from build123d import *

# Parameters (mm, degrees)
BOX007_W     = 7
BOX007_H     = 4
BOX007_DEPTH = 6
BOX002_W     = 30.1
BOX002_H     = 23.1
BOX002_DEPTH = 4
BOX003_W     = 12
BOX003_H     = 7
BOX003_DEPTH = 10
BOX001_W     = 40
BOX001_H     = 3
BOX001_DEPTH = 12
BOX004_W     = 4
BOX004_H     = 4
BOX004_DEPTH = 6
BOX005_W     = 4
BOX005_H     = 4
BOX005_DEPTH = 6
BOX008_W     = 30
BOX008_H     = 30
BOX008_DEPTH = 3
BOX006_W     = 19
BOX006_H     = 4
BOX006_DEPTH = 5


with BuildPart() as cube007:
    # Box007 → Box007 (new body)
    with BuildSketch(Plane(origin=(25, 1, 3), x_dir=(1, 0, 0), z_dir=(0, 0, 1))):
        with Locations((3.5, 2)):
            Rectangle(BOX007_W, BOX007_H)
    extrude(amount=BOX007_DEPTH)


with BuildPart() as cube002:
    # Box002 → Box002 (new body)
    with BuildSketch(Plane(origin=(7, 1, 3), x_dir=(1, 0, 0), z_dir=(0, 0, 1))):
        with Locations((15.05, 11.55)):
            Rectangle(BOX002_W, BOX002_H)
    extrude(amount=BOX002_DEPTH)


with BuildPart() as cube003:
    # Box003 → Box003 (new body)
    with BuildSketch(Plane(origin=(13, -4, 1), x_dir=(1, 0, 0), z_dir=(0, 0, 1))):
        with Locations((6, 3.5)):
            Rectangle(BOX003_W, BOX003_H)
    extrude(amount=BOX003_DEPTH)


with BuildPart() as cube001:
    # Box001 → Box001 (new body)
    with BuildSketch(Plane.XY):
        with Locations((20, 1.5)):
            Rectangle(BOX001_W, BOX001_H)
    extrude(amount=BOX001_DEPTH)


with BuildPart() as cube004:
    # Box004 → Box004 (new body)
    with BuildSketch(Plane(origin=(23, 22, 3), x_dir=(1, 0, 0), z_dir=(0, 0, 1))):
        with Locations((2, 2)):
            Rectangle(BOX004_W, BOX004_H)
    extrude(amount=BOX004_DEPTH)


with BuildPart() as cube005:
    # Box005 → Box005 (new body)
    with BuildSketch(Plane(origin=(4, 22, 3), x_dir=(1, 0, 0), z_dir=(0, 0, 1))):
        with Locations((2, 2)):
            Rectangle(BOX005_W, BOX005_H)
    extrude(amount=BOX005_DEPTH)


with BuildPart() as cut001:
    # Box008 → Box008 (new body)
    with BuildSketch(Plane.XY):
        with Locations((15, 15)):
            Rectangle(BOX008_W, BOX008_H)
    extrude(amount=BOX008_DEPTH)

    # Fusion001: union Cube001, Cube004, Cube005
    add(cube001.part)
    add(cube004.part)
    add(cube005.part)

    # Cut: cut Cube003
    add(cube003.part, mode=Mode.SUBTRACT)

    # Cut001: cut Cube002
    add(cube002.part, mode=Mode.SUBTRACT)


with BuildPart() as obj1:
    # Box006 → Box006 (new body)
    with BuildSketch(Plane(origin=(7, 1, 0), x_dir=(1, 0, 0), z_dir=(0, 0, 1))):
        with Locations((9.5, 2)):
            Rectangle(BOX006_W, BOX006_H)
    extrude(amount=BOX006_DEPTH)

    # Fusion002: union Cut001
    add(cut001.part)

    # Cut002: cut Cube007
    add(cube007.part, mode=Mode.SUBTRACT)


with BuildPart() as obj1_1:
    # Cut002 placement: moved
    add(obj1.part.moved(Location((113, -95, 26.4))))


solid = obj1_1.part
Read the model definition and answer for the solid it produces. Units are mm, in the model's axes. A direction names the side the tool comes from. Give positions to 0.01 mm unless a question says otherwise; leave off trailing zeros. Loops run counter-clockwise (first coordinate to the right, second up) from the corner with the lowest first, then second, coordinate; pieces in that order, holes last. Notation, with made-up numbers: (10.5, 70) -> (64.5, 70) arc R4 ccw to (64.5, 74) -> close; hole circle Ø4 at (34, -28). An arc over 180 degrees is marked (long way). Use a Markdown table: item, result.
Q1. Each of these flat-tipped pins is pushed along its axis until it touches: pin 1 (1.2 mm diameter, centred on y = -71.5, z = 32, fed in from -X); pin 2 (1 mm diameter, centred on x = 123, z = 32.5, fed in from +Y); pin 3 (4 mm diameter, centred on y = -88, z = 33, fed in from -X); pin 4 (3 mm diameter, centred on x = 134, z = 29.5, fed in from -Y). Where does it stop, or does it pass through?
Solved:
| item | result |
|---|---|
| pin 1 | stops at x = 117 |
| pin 2 | stops at y = -94 |
| pin 3 | passes through |
| pin 4 | stops at y = -94 |
Q2. Section A-A, the plane x = 130.5 is taken. Determine the outline of the cut face in (y, z).
Solved:
| item | result |
|---|---|
| outline | (-95, 26.4) -> (-65, 26.4) -> (-65, 29.4) -> (-90, 29.4) -> (-90, 31.4) -> (-94, 31.4) -> (-94, 27.4) -> (-95, 27.4) -> close; (-95, 37.4) -> (-92, 37.4) -> (-92, 38.4) -> (-95, 38.4) -> close |
Q3. A tool of negligible diameter and unlimited length cuts with its end or side. For faces 5 (the face through (141, -93, 35.4)), 6 (the face through (138, -69, 32)), 7 (the face through (148, -93, 33.4)), from which of +Z, -Z, +X, -X, +Y, -Y can it reach the whole face along a straight path? Write none if from no direction.
Solved:
| item | result |
|---|---|
| face 5 | none |
| face 6 | +Z, +X, -X, +Y |
| face 7 | +Y |
Q4. Section D-D, the plane x = 142 is taken. Determine the outline of the cut face in (y, z), then the cut area to 3 significant figures.
Solved:
| item | result |
|---|---|
| outline | (-95, 26.4) -> (-65, 26.4) -> (-65, 29.4) -> (-94, 29.4) -> (-94, 35.4) -> (-92, 35.4) -> (-92, 38.4) -> (-95, 38.4) -> close |
| area | 105 mm^2 |
Q5. Section C-C, the plane z = 34.5 is taken. Determine the outline of the cut face in (x, y).
Solved:
| item | result |
|---|---|
| outline | (113, -95) -> (126, -95) -> (126, -92) -> (113, -92) -> close; (117, -73) -> (121, -73) -> (121, -69) -> (117, -69) -> close; (136, -73) -> (140, -73) -> (140, -69) -> (136, -69) -> close; (138, -95) -> (153, -95) -> (153, -92) -> (145, -92) -> (145, -94) -> (138, -94) -> close |
Q6. Find the intervals of material crossed by line 1 along Z through (x, y) = (139, -92.75); line 2 along Z through (x, y) = (132, -76.25); line 3 along X through (y, z) = (-86, 28), in increasing order.
Solved:
| item | result |
|---|---|
| line 1 | z = 26.4 to 29.4, 35.4 to 38.4 |
| line 2 | z = 26.4 to 29.4 |
| line 3 | x = 113 to 143 |
Q7. Determine the mould class of faces 1 (the face through (126, -94.2, 33.4)), 2 (the face through (119, -73, 32)), 3 (the face through (132, -93, 37.4)), 4 (the face through (138, -71, 35.4)) for opening direction Z: pulls with the +Z half, pulls with the -Z half, needs draft (parallel to the pull), parting line crosses it, or undercut.
Solved:
| item | result |
|---|---|
| face 1 | undercut |
| face 2 | needs draft |
| face 3 | undercut |
| face 4 | pulls with the +Z half |
Q8. Section B-B, the plane y = -91 is taken. Determine the outline of the cut face in (x, z).
Solved:
| item | result |
|---|---|
| outline | (113, 26.4) -> (143, 26.4) -> (143, 29.4) -> (138, 29.4) -> (138, 31.4) -> (120, 31.4) -> (120, 29.4) -> (113, 29.4) -> close |
